```python
from build123d import *

# Parameters (mm, degrees)
F1_DEPTH = 3.175


with BuildPart() as f1:
    # F0 (on Front) → F1 (new body)
    with BuildSketch(Plane.XZ):
        with BuildLine():
            Line((94.2812450191, 0), (0, 0))
            ThreePointArc((0, 0), (-16.002, -16.002), (0, -32.004))
            ThreePointArc((0, -32.004), (5.7669601924, -30.1895691641), (9.4561357565, -25.4))
            Line((9.4561357565, -25.4), (60.198, -25.4))
            Line((60.198, -25.4), (60.198, -35.052))
            ThreePointArc((60.198, -35.052), (63.373, -35.8398051697), (66.548, -35.052))
            Line((66.548, -35.052), (66.548, -31.75))
            Line((66.548, -31.75), (123.3573333658, -31.75))
            ThreePointArc((123.3573333658, -31.75), (133.627989797, -29.808331099), (142.4810210729, -24.2513266114))
            Line((142.4810210729, -24.2513266114), (161.798, -6.35))
            Line((161.798, -6.35), (107.4487924851, -0.6844598091))
            ThreePointArc((107.4487924851, -0.6844598091), (100.873907446, -0.1712303847), (94.2812450191, 0))
        make_face()
    extrude(amount=F1_DEPTH)

    # F3: sweep along a path in F3_path
    with BuildLine(Plane(origin=(66.548, -3.175, -31.75), x_dir=(0, 0, -1), z_dir=(0, 1, 0))) as f3_path:
        Line((0, 0), (0, -56.8093333658))
        ThreePointArc((0, -56.8093333658), (-1.941668901, -67.079989797), (-7.4986733886, -75.9330210729))
        Line((-7.4986733886, -75.9330210729), (-25.4, -95.25))
    # F2 (on face) → F3 (sweep, cut)
    with BuildSketch(Plane.YZ.offset(66.548)):
        Polygon((-3.175, -31.75), (-1.651, -31.75), (-3.175, -20.9061765431), align=None)
    sweep(path=f3_path.line, mode=Mode.SUBTRACT)

    # F5: sweep along a path in F5_path
    with BuildLine(Plane(origin=(123.3573333658, 0, -31.75), x_dir=(0, 0, -1), z_dir=(0, 1, 0))) as f5_path:
        Line((0, 56.8093333658), (0, 0))
        ThreePointArc((0, 0), (-1.941668901, -10.2706564312), (-7.4986733886, -19.1236877071))
        Line((-7.4986733886, -19.1236877071), (-25.4, -38.4406666342))
    # F4 (on face) → F5 (sweep, cut)
    with BuildSketch(Plane.YZ.offset(66.548)):
        Polygon((0, -20.9061765431), (-1.524, -31.75), (0, -31.75), align=None)
    sweep(path=f5_path.line, mode=Mode.SUBTRACT)


solid = f1.part
```
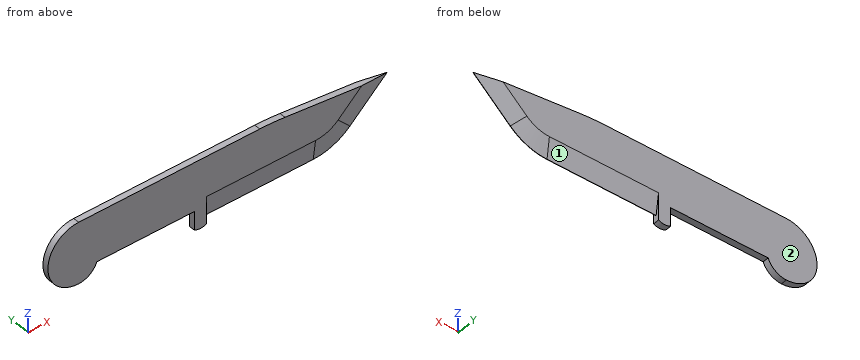
Design review of the part built by this model. Coordinates are the model's own, in mm. Face numbers are marked on the shaded views. A direction names the side the tool comes from. Give positions to 0.01 mm unless a question says otherwise; leave off trailing zeros. Loops run counter-clockwise (first coordinate to the right, second up) from the corner with the lowest first, then second, coordinate; pieces in that order, holes last. Notation, with made-up numbers: M 39,-38 L 81,-38 A7 ccw 81,-32 Z; hole C 29,-11.5 d11. An arc over 180 degrees is marked long. Return JSON: item names as keys, results as strings. Group by question number.
Item 1: Insertion check: pin 1 Ø1 at (x, y) = (15, -2.5) entering from -Z; pin 2 Ø2 at (x, z) = (36, -26.5) entering from -Y; pin 3 Ø1.5 at (x, z) = (126.5, -23.5) entering from +Y. Each pin has a flat end and moves straight along its axis. Give the tip position at first contact, or say it passes through.
Item 2: For probe 1 along Z at (x, y) = (32, -1); probe 2 along Y at (x, z) = (99.5, -22); probe 3 along Z at (x, y) = (3.5, -0.95), list the stretches that pass through material, from the lowest coordinate up.
Item 3: We need section B-B (y = -0.8). Give the boundary of the cut face in (x, z), and give its area (3 significant figures).
Item 4: We need section C-C (x = 119.5). Give the boundary of the cut face in (y, z) (3 decimals).
Item 5: We need section A-A (x = 88). Give the boundary of the cut face in (y, z) (3 decimals), and give its area (3 significant figures).
Item 6: Tool access review of the marked faces 1 and 2: name each direction out of +Z, -Z, +X, -X, +Y, -Y from which nothing blocks a thin tool from reaching the whole face with its end or side.
Output:
{
 "1": {"pin 1": "stops at z = -25.4", "pin 2": "passes through", "pin 3": "stops at y = -0.29"},
 "2": {"probe 1": "z = -25.4 to 0", "probe 2": "y = -3.02 to -0.15", "probe 3": "z = -31.38 to 0"},
 "3": {"outline": "M 0,-32 A10.07 ccw 9.46,-25.4 L 60.2,-25.4 L 60.2,-35.05 A6.79 ccw 66.55,-35.05 L 66.55,-26.6 L 123.36,-26.6 A22.98 ccw 138.98,-20.47 L 154.99,-5.64 L 107.45,-0.68 A127 ccw 94.28,0 L 0,0 A16 ccw Z", "area": "4,150 mm^2"},
 "4": {"outline": "M -3.175,-20.906 L -1.651,-31.75 L -1.524,-31.75 L 0,-20.906 L 0,-1.941 L -3.175,-1.941 Z"},
 "5": {"outline": "M -3.175,-20.906 L -1.651,-31.75 L -1.524,-31.75 L 0,-20.906 L 0,0 L -3.175,0 Z", "area": "84.3 mm^2"},
 "6": {"face 1": "-Z, +X, +Y", "face 2": "+Z, -Z, +X, -X, +Y"}
}
